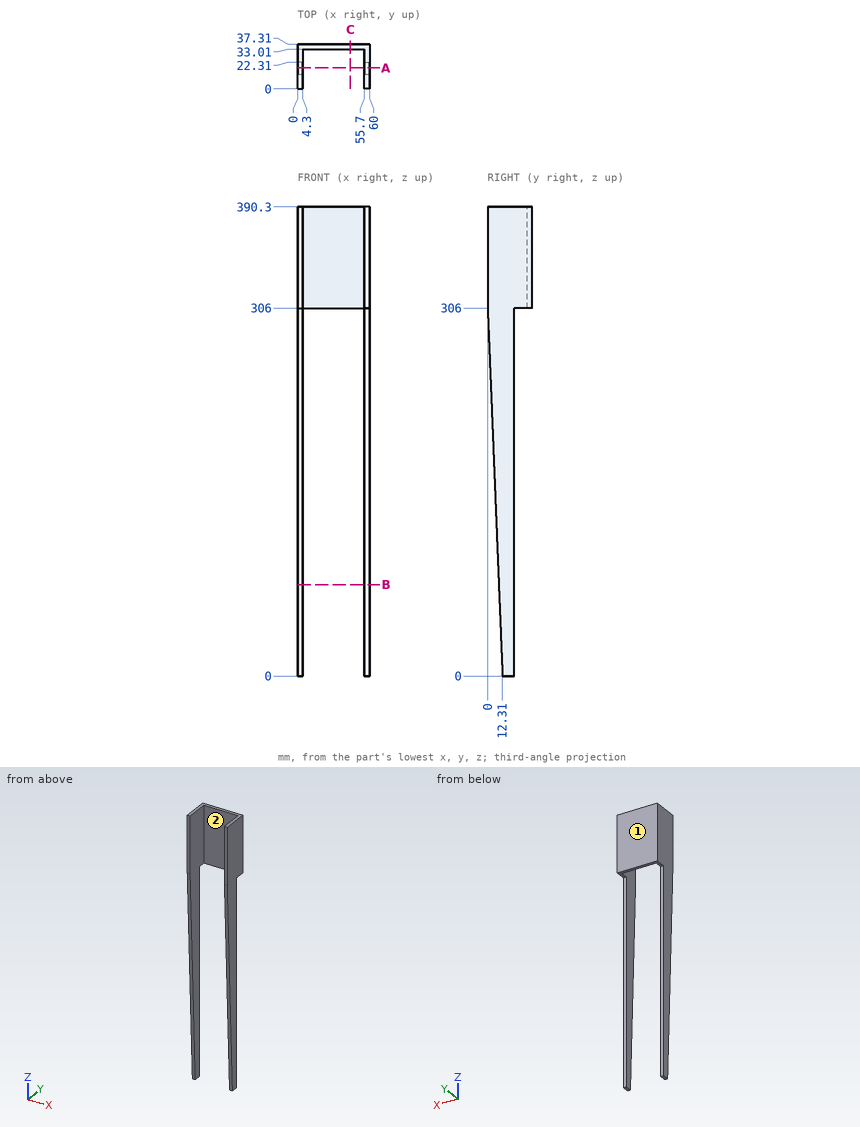
For this review, use the dimensioned drawing (mm, ordinates from the lowest corner) and the shaded views. Give positions to 0.01 mm unless a question says otherwise; leave off trailing zeros. Order: outer loops, then holes, each group sorted by start corner. A loop starts at its lowest first (then second) coordinate and runs counter-clockwise, first axis right, second up.
1) Insertion check: pin 1 (12 mm diameter, centred on x = 34.5, y = 27.5, fed in from +Z); pin 2 (7.5 mm diameter, centred on x = 42.5, y = 29, fed in from -Z); pin 3 (10 mm diameter, centred on x = 10.5, z = 303.5, fed in from -Y); pin 4 (1.3 mm diameter, centred on x = 57.5, z = 157.5, fed in from +Y). Each pin has a flat end and moves straight along its axis. Give the tip position at first contact, or say it passes through.
2) Wall thickness on line 1 (X direction, y = 18.5, z = 298); line 2 (Y direction, x = 35, z = 350); line 3 (Z direction, x = 4, y = 28): over which ranges is each line inside the solid? List them lowest first.
3) Take a section at C-C (x = 44). Give the boundary of the cut face in (y, z), then the cut area to 3 significant figures.
4) Take a section at A-A (y = 17.5). Give the boundary of the cut face in (x, z).
5) The part is to be moulded in two halves that separate along X. For the marked faces 1 and 2, say which applies: released by +X, released by -X, zero draft, split by the parting line, or undercut.
6) Take a section at B-B (z = 76). Give the boundary of the cut face in (x, y), then the cut area to 3 significant figures.
Derived:
1. pin 1: stops at z = 390.3
1. pin 2: passes through
1. pin 3: stops at y = 33.01
1. pin 4: stops at y = 22.31
2. line 1: x = 0 to 4.3, 55.7 to 60
2. line 2: y = 33.01 to 37.31
2. line 3: z = 306 to 390.3
3. outline: (33.01, 306) - (37.31, 306) - (37.31, 390.3) - (33.01, 390.3) - close
3. area: 362 mm2
4. outline: (0, 0) - (4.3, 0) - (4.3, 390.3) - (0, 390.3) - close; (55.7, 0) - (60, 0) - (60, 390.3) - (55.7, 390.3) - close
5. face 1: zero draft
5. face 2: undercut
6. outline: (0, 9.25) - (4.3, 9.25) - (4.3, 22.31) - (0, 22.31) - close; (55.7, 9.25) - (60, 9.25) - (60, 22.31) - (55.7, 22.31) - close
6. area: 112 mm2
